```python
from build123d import *

# Parameters (mm, degrees)
SKETCH2_W           = 200
SKETCH2_H           = 185
BOSS_EXTRUDE1_DEPTH = 5
SKETCH3_W           = 5.5
SKETCH3_H           = 50
SKETCH3_R           = 1.5
CUT_EXTRUDE1_DEPTH  = 137.313058802
SKETCH4_R           = 1.5
CUT_EXTRUDE3_DEPTH  = 137.313058802
FILLET1_R           = 8


with BuildPart() as part:
    # Sketch2 → Boss-Extrude1 (new body)
    with BuildSketch(Plane(origin=(0, 0, 0), x_dir=(1, 0, 0), z_dir=(0, 1, 0))):
        Rectangle(SKETCH2_W, SKETCH2_H)
        with BuildLine():
            Line((-95, 55.5), (-95, 82.5))
            ThreePointArc((-95, 82.5), (-93.5, 84), (-92, 82.5))
            Line((-92, 82.5), (-92, 55.5))
            ThreePointArc((-92, 55.5), (-93.5, 54), (-95, 55.5))
        make_face(mode=Mode.SUBTRACT)
        with BuildLine():
            Line((95, 55.5), (95, 82.5))
            ThreePointArc((95, 82.5), (93.5, 84), (92, 82.5))
            Line((92, 82.5), (92, 55.5))
            ThreePointArc((92, 55.5), (93.5, 54), (95, 55.5))
        make_face(mode=Mode.SUBTRACT)
        with BuildLine():
            Line((95, -55.5), (95, -82.5))
            ThreePointArc((95, -82.5), (93.5, -84), (92, -82.5))
            Line((92, -82.5), (92, -55.5))
            ThreePointArc((92, -55.5), (93.5, -54), (95, -55.5))
        make_face(mode=Mode.SUBTRACT)
        with BuildLine():
            Line((-95, -55.5), (-95, -82.5))
            ThreePointArc((-95, -82.5), (-93.5, -84), (-92, -82.5))
            Line((-92, -82.5), (-92, -55.5))
            ThreePointArc((-92, -55.5), (-93.5, -54), (-95, -55.5))
        make_face(mode=Mode.SUBTRACT)
    extrude(amount=BOSS_EXTRUDE1_DEPTH)

    # Sketch3 → Cut-Extrude1 (cut, through all)
    with BuildSketch(Plane(origin=(0, 5, 0), x_dir=(1, 0, 0), z_dir=(0, 1, 0))):
        with BuildLine():
            Line((-82.5, 42.5), (-42.5, 42.5))
            ThreePointArc((-42.5, 42.5), (-40, 45), (-42.5, 47.5))
            Line((-42.5, 47.5), (-82.5, 47.5))
            ThreePointArc((-82.5, 47.5), (-85, 45), (-82.5, 42.5))
        make_face()
        with BuildLine():
            ThreePointArc((-42.5, -42.5), (-40, -45), (-42.5, -47.5))
            Line((-42.5, -47.5), (-82.5, -47.5))
            ThreePointArc((-82.5, -47.5), (-85, -45), (-82.5, -42.5))
            Line((-82.5, -42.5), (-42.5, -42.5))
        make_face()
        with Locations((-87.25, 0)):
            Rectangle(SKETCH3_W, SKETCH3_H)
        with Locations((-51.75, 0)):
            Rectangle(SKETCH3_W, SKETCH3_H)
        with Locations(Location((-90, -30, 0), (0, 0, 270))):
            Circle(SKETCH3_R)
        with Locations(Location((-90, 30, 0), (0, 0, 90))):
            Circle(SKETCH3_R)
        with Locations(Location((-35, -30, 0), (0, 0, 90))):
            Circle(SKETCH3_R)
        with Locations(Location((-35, 30, 0), (0, 0, 270))):
            Circle(SKETCH3_R)
    extrude(amount=-CUT_EXTRUDE1_DEPTH, mode=Mode.SUBTRACT)

    # Sketch4 → Cut-Extrude3 (cut, through all)
    with BuildSketch(Plane(origin=(0, 5, 0), x_dir=(1, 0, 0), z_dir=(0, 1, 0))):
        with Locations(Location((8, 46.935, 0), (0, 0, 270))):
            Circle(SKETCH4_R)
        with Locations(Location((52, 46.935, 0), (0, 0, 90))):
            Circle(SKETCH4_R)
        with Locations(Location((6, -46.935, 0), (0, 0, 270))):
            Circle(SKETCH4_R)
        with Locations(Location((54, -46.935, 0), (0, 0, 90))):
            Circle(SKETCH4_R)
        with BuildLine():
            Line((71.5, -60), (71.5, 60))
            ThreePointArc((71.5, 60), (74, 62.5), (76.5, 60))
            Line((76.5, 60), (76.5, -60))
            ThreePointArc((76.5, -60), (74, -62.5), (71.5, -60))
        make_face()
        with BuildLine():
            Line((-16.5, -60), (-16.5, 60))
            ThreePointArc((-16.5, 60), (-14, 62.5), (-11.5, 60))
            Line((-11.5, 60), (-11.5, -60))
            ThreePointArc((-11.5, -60), (-14, -62.5), (-16.5, -60))
        make_face()
        with BuildLine():
            Line((0, 69.435), (60, 69.435))
            ThreePointArc((60, 69.435), (62.5, 66.935), (60, 64.435))
            Line((60, 64.435), (0, 64.435))
            ThreePointArc((0, 64.435), (-2.5, 66.935), (0, 69.435))
        make_face()
        with BuildLine():
            Line((0, -69.435), (60, -69.435))
            ThreePointArc((60, -69.435), (62.5, -66.935), (60, -64.435))
            Line((60, -64.435), (0, -64.435))
            ThreePointArc((0, -64.435), (-2.5, -66.935), (0, -69.435))
        make_face()
    extrude(amount=-CUT_EXTRUDE3_DEPTH, mode=Mode.SUBTRACT)

    # Fillet1
    fillet1_edges = [part.edges().sort_by_distance(p)[0] for p in [
        (100, 2.5, 92.5),
        (-100, 2.5, 92.5),
        (-100, 2.5, -92.5),
        (100, 2.5, -92.5),
    ]]
    fillet(fillet1_edges, radius=FILLET1_R)


solid = part.part
```
Geometry: final body of the model. Coordinates: model frame, mm. A direction names the side the tool comes from. Give positions to 0.01 mm unless a question says otherwise; leave off trailing zeros. Loops run counter-clockwise (first coordinate to the right, second up) from the corner with the lowest first, then second, coordinate; pieces in that order, holes last. Notation, with made-up numbers: (-10.5, 71) - (9.5, 71) arc R24 cw to (9.5, 89) - close; hole circle Ø9 at (22.25, 53). An arc over 180 degrees is marked (long way). Answer as CSV lines item,"result". Start each with the question number.
(1) Section query A-A (z = 80). Output: boundary loops of the cut face in (x, y).
(2) Reachability of faces 1 (the face through (-1, 0, -1)), 2 (the face through (-90, 3, 0)) from +Z, -Z, +X, -X, +Y, -Y: full face, straight path, thin tool, end or side. Return the list, or none.
(3) Section query C-C (z = -7). Output: boundary loops of the cut face in (x, y).
(4) Section query D-D (y = 0.95). Give the number of separate pieces and of enclosed holes in the cut face, and give its area (3 significant figures).
(5) Section query B-B (x = -61.5). Output: boundary loops of the cut face in (y, z).
(6) Ray query, line 1 along Z through (x, y) = (1, 1.4) (3 decimals); line 2 along X through (y, z) = (2.8, -18); line 3 along X through (y, z) = (2.25, -49). Return the intervals inside material, ascending. Write a range as [from, to].
(7) Mould query, pull axis Z, two halves, no side actions, for faces 3 (the face through (100, 2, 1)), 4 (the face through (30, 3, 64.435)), 5 (the face through (-97.719, 2.535, 90.094)). Classes: +Z half, -Z half, draft (parallel to the pull), parting line (faces both ways), or undercut.
(8) Pin query (flat end, axial travel): P1, Ø2.5, axis at x = -90, z = -30, coming from the +Y side. Return the tip coordinate at first contact, or that it passes through.
Worked answers:
1,outline,"(-100, 0) - (-95, 0) - (-95, 5) - (-100, 5) - close; (-92, 0) - (92, 0) - (92, 5) - (-92, 5) - close; (95, 0) - (100, 0) - (100, 5) - (95, 5) - close"
2,face 1,"+Z, -Z, +X, -X, -Y"
2,face 2,"+Y, -Y"
3,outline,"(-100, 0) - (-90, 0) - (-90, 5) - (-100, 5) - close; (-84.5, 0) - (-54.5, 0) - (-54.5, 5) - (-84.5, 5) - close; (-49, 0) - (-16.5, 0) - (-16.5, 5) - (-49, 5) - close; (-11.5, 0) - (71.5, 0) - (71.5, 5) - (-11.5, 5) - close; (76.5, 0) - (100, 0) - (100, 5) - (76.5, 5) - close"
4,separate pieces,"1"
4,enclosed holes,"20"
4,area,"33,700 mm^2"
5,outline,"(0, -92.5) - (5, -92.5) - (5, -47.5) - (0, -47.5) - close; (0, -42.5) - (5, -42.5) - (5, 42.5) - (0, 42.5) - close; (0, 47.5) - (5, 47.5) - (5, 92.5) - (0, 92.5) - close"
6,line 1,"z = [-92.5, -69.435], [-64.435, 64.435], [69.435, 92.5]"
6,line 2,"x = [-100, -90], [-84.5, -54.5], [-49, -16.5], [-11.5, 71.5], [76.5, 100]"
6,line 3,"x = [-100, -16.5], [-11.5, 71.5], [76.5, 100]"
7,face 3,"draft"
7,face 4,"undercut"
7,face 5,"+Z half"
8,P1,"passes through"
